from build123d import *

# Parameters (mm, degrees)
BOSS_EXTRUDE1_DEPTH = 6


with BuildPart() as part:
    # Sketch1 → Boss-Extrude1 (new body)
    with BuildSketch(Plane.XY):
        with BuildLine():
            Line((12.7, 0), (241.3, 0))
            ThreePointArc((241.3, 0), (250.280256121, 3.719743879), (254, 12.7))
            Line((254, 12.7), (254, 51.507746743))
            ThreePointArc((254, 51.507746743), (252.641048665, 63.179195107), (248.636901303, 74.226197394))
            Line((248.636901303, 74.226197394), (215.600193669, 140.299612663))
            ThreePointArc((215.600193669, 140.299612663), (210.917753467, 145.423265266), (204.240968343, 147.32))
            Line((204.240968343, 147.32), (49.759031657, 147.32))
            ThreePointArc((49.759031657, 147.32), (43.082246533, 145.423265266), (38.399806331, 140.299612663))
            Line((38.399806331, 140.299612663), (5.363098697, 74.226197394))
            ThreePointArc((5.363098697, 74.226197394), (1.358951335, 63.179195107), (0, 51.507746743))
            Line((0, 51.507746743), (0, 12.7))
            ThreePointArc((0, 12.7), (3.719743879, 3.719743879), (12.7, 0))
        make_face()
        with BuildLine():
            Line((40.939806331, 81.879612663), (53.639806331, 107.279612663))
            ThreePointArc((53.639806331, 107.279612663), (58.322246533, 112.403265266), (64.999031657, 114.3))
            Line((64.999031657, 114.3), (189.000968343, 114.3))
            ThreePointArc((189.000968343, 114.3), (195.677753467, 112.403265266), (200.360193669, 107.279612663))
            Line((200.360193669, 107.279612663), (213.060193669, 81.879612663))
            ThreePointArc((213.060193669, 81.879612663), (212.504233609, 69.523214876), (201.700968343, 63.5))
            Line((201.700968343, 63.5), (52.299031657, 63.5))
            ThreePointArc((52.299031657, 63.5), (41.495766391, 69.523214876), (40.939806331, 81.879612663))
        make_face(mode=Mode.SUBTRACT)
    extrude(amount=BOSS_EXTRUDE1_DEPTH)


solid = part.part
The listing builds one solid part. Answer for the finished solid, in the listing's coordinates (mm). A direction names the side the tool comes from. Give positions to 0.01 mm unless a question says otherwise; leave off trailing zeros. Loops run counter-clockwise (first coordinate to the right, second up) from the corner with the lowest first, then second, coordinate; pieces in that order, holes last.
Item 1: A tool of negligible diameter and unlimited length cuts with its end or side. For faces 1 (the flat face through (47, 94, 3)), 2 (the cylindrical face through (250.18, 3.62, 2.96)), from which of +Z, -Z, +X, -X, +Y, -Y can it reach the whole face along a straight path? Write none if from no direction.
Derived:
face 1: +Z, -Z
face 2: +Z, -Z, +X, -Y
Item 2: Find the intervals of material crossed by line 1 along Y through (x, z) = (149, 3.1); line 2 along Y through (x, z) = (201.5, 1.3); line 3 along X through (y, z) = (77, 2.6), in increasing order.
Derived:
line 1: y = 0 to 63.5, 114.3 to 147.32
line 2: y = 0 to 63.5, 105 to 147.32
line 3: x = 6.75 to 39.62, 214.38 to 247.25
Item 3: A cutting plane is placed at D-D (x = 228). Give the vertices of the cut face in (y, z), then the cut area to 3 significant figures.
Derived:
outline: (0, 0) - (115.5, 0) - (115.5, 6) - (0, 6) - close
area: 693 mm2
Item 4: Determine the mould class of faces 3 (the flat face through (125, 58, 0)), 4 (the cylindrical face through (41.59, 69.37, 2.96)), 5 (the cylindrical face through (3.62, 3.82, 2.96)) for opening direction X: +X half, -X half, draft (parallel to the pull), parting line (faces both ways), or undercut.
Derived:
face 3: draft
face 4: undercut
face 5: -X half
Item 5: A cutting plane is placed at A-A (x = 120.5). Give the vertices of the cut face in (y, z), then the cut area to 3 significant figures.
Derived:
outline: (0, 0) - (63.5, 0) - (63.5, 6) - (0, 6) - close; (114.3, 0) - (147.32, 0) - (147.32, 6) - (114.3, 6) - close
area: 579 mm2
Item 6: A cutting plane is placed at B-B (y = 94). Give the vertices of the cut face in (x, z), then the cut area to 3 significant figures.
Derived:
outline: (15.25, 0) - (47, 0) - (47, 6) - (15.25, 6) - close; (207, 0) - (238.75, 0) - (238.75, 6) - (207, 6) - close
area: 381 mm2
Item 7: This flat-tipped pin is pushed along its axis until it touches: pin 1 Ø8 at (x, y) = (40.5, 78.5) entering from -Z. Where does it stop, or does it pass through?
Derived:
pin 1: stops at z = 0
Item 8: A cutting plane is placed at C-C (z = 1). Give the vertices of the cut face in (x, y).
Derived:
outline: (0, 12.7) arc R12.7 ccw to (12.7, 0) - (241.3, 0) arc R12.7 ccw to (254, 12.7) - (254, 51.51) arc R50.8 ccw to (248.64, 74.23) - (215.6, 140.3) arc R12.7 ccw to (204.24, 147.32) - (49.76, 147.32) arc R12.7 ccw to (38.4, 140.3) - (5.36, 74.23) arc R50.8 ccw to (0, 51.51) - close; hole (40.94, 81.88) arc R12.7 ccw to (52.3, 63.5) - (201.7, 63.5) arc R12.7 ccw to (213.06, 81.88) - (200.36, 107.28) arc R12.7 ccw to (189, 114.3) - (65, 114.3) arc R12.7 ccw to (53.64, 107.28) - close
